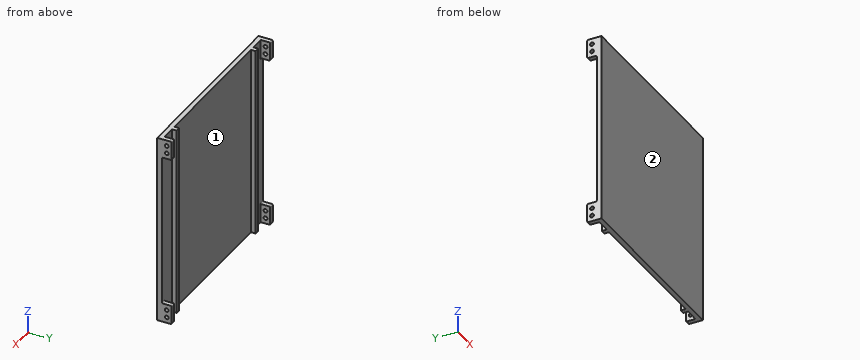
from build123d import *

# Parameters (mm, degrees)
SKETCH1_W            = 200
SKETCH1_H            = 5
BOSS_EXTRUDE1_DEPTH  = 100
SKETCH2_W            = 5
SKETCH2_H            = 200
BOSS_EXTRUDE2_DEPTH  = 5
SKETCH3_W            = 5
SKETCH3_H            = 20
BOSS_EXTRUDE3_DEPTH  = 10
SKETCH4_R            = 2
CUT_EXTRUDE1_DEPTH   = 10
FILLET1_R            = 1
FILLET1_OF_MIRROR1_R = 1


with BuildPart() as part:
    # Sketch1 → Boss-Extrude1 (new, symmetric)
    with BuildSketch(Plane.XY):
        with Locations((0, -2.5)):
            Rectangle(SKETCH1_W, SKETCH1_H)
    extrude(amount=BOSS_EXTRUDE1_DEPTH, both=True)

    # Sketch2 → Boss-Extrude2 (add)
    with BuildSketch(Plane(origin=(0, 0, 0), x_dir=(1, 0, 0), z_dir=(0, 1, 0))):
        with Locations((-78, 0)):
            Rectangle(SKETCH2_W, SKETCH2_H)
        with Locations((78, 0)):
            Rectangle(SKETCH2_W, SKETCH2_H)
    extrude(amount=BOSS_EXTRUDE2_DEPTH)

    # Sketch3 → Boss-Extrude3 (add)
    with BuildSketch(Plane(origin=(0, 0, 0), x_dir=(1, 0, 0), z_dir=(0, 1, 0))):
        with Locations((-97.5, -90)):
            Rectangle(SKETCH3_W, SKETCH3_H)
        with Locations((-97.5, 90)):
            Rectangle(SKETCH3_W, SKETCH3_H)
    boss_extrude3 = extrude(amount=BOSS_EXTRUDE3_DEPTH)

    # Sketch4 → Cut-Extrude1 (cut)
    with BuildSketch(Plane.ZY.offset(100)):
        with Locations((-86, 5)):
            Circle(SKETCH4_R)
        with Locations((-94, 5)):
            Circle(SKETCH4_R)
        with Locations((94, 5)):
            Circle(SKETCH4_R)
        with Locations((86, 5)):
            Circle(SKETCH4_R)
        with Locations((-86, 5)):
            Circle(SKETCH4_R)
        with Locations((-94, 5)):
            Circle(SKETCH4_R)
    cut_extrude1 = extrude(amount=-CUT_EXTRUDE1_DEPTH, mode=Mode.SUBTRACT)

    # Fillet1
    fillet1_edges = [part.edges().sort_by_distance(p)[0] for p in [
        (-97.5, 0, 80),
        (-97.5, 10, 100),
        (-97.5, 10, 80),
        (-97.5, 0, -80),
        (-97.5, 10, -100),
        (-97.5, 10, -80),
    ]]
    fillet(fillet1_edges, radius=FILLET1_R)

    # Mirror1: Boss-Extrude3, Cut-Extrude1 across plane
    add(boss_extrude3.mirror(Plane(origin=(0, 0, 0), x_dir=(0, 0, 1), z_dir=(1, 0, 0))))
    add(cut_extrude1.mirror(Plane(origin=(0, 0, 0), x_dir=(0, 0, 1), z_dir=(1, 0, 0))), mode=Mode.SUBTRACT)

    # Fillet1 of Mirror1
    fillet1_of_mirror1_edges = [part.edges().sort_by_distance(p)[0] for p in [
        (97.5, 0, 80),
        (97.5, 10, 100),
        (97.5, 10, 80),
        (97.5, 0, -80),
        (97.5, 10, -100),
        (97.5, 10, -80),
    ]]
    fillet(fillet1_of_mirror1_edges, radius=FILLET1_OF_MIRROR1_R)


solid = part.part
Input: part model. Units: mm. Frame: model coordinates. Face numbers are marked on the shaded views. Coordinates: 2 decimals unless noted, no trailing zeros. Order: outer loops, then holes, each group sorted by start corner. A loop starts at its lowest first (then second) coordinate and runs counter-clockwise, first axis right, second up. Notation, with made-up numbers: M -6.75,18.25 L 45.25,18.25 A22 cw 45.25,29.25 Z; hole C -7.75,48 d6. An arc over 180 degrees is marked long. Write item = value, one per line. Start each with the question number.
(1) Pull-direction query (X, two-part tool) for the marked faces 1 and 2; classes: released by +X, released by -X, zero draft, split by the parting line, or undercut.
(2) First-contact query: P1, Ø3.5, axis at y = 5, z = 94, coming from the +X side; P2, Ø2.5, axis at y = 5, z = 94, coming from the -X side; P3, Ø6, axis at x = 15, z = -64.5, coming from the +Y side. Flat tips, straight axial feed; report the tip coordinate or a pass-through.
(3) Section C-C on x = 78. Output: boundary loops of the cut face in (y, z), and give its area (3 significant figures).
(4) Line query: line 1 along X through (y, z) = (2, -82); line 2 along Z through (x, y) = (97.65, 5); line 3 along X through (y, z) = (0.25, 54). Output: solid intervals per line, ascending. Write a range as [from, to].
(5) Section A-A on z = 10. Output: boundary loops of the cut face in (x, y), and give its area (3 significant figures).
(6) Section B-B on x = 53. Output: boundary loops of the cut face in (y, z).
Result set:
q1.face_1 = undercut
q1.face_2 = zero draft
q2.P1 = 80.5
q2.P2 = -80.5
q2.P3 = 0
q3.outline = M -5,-100 L 5,-100 L 5,100 L -5,100 Z
q3.area = 2,000 mm²
q4.line_1 = [-100, -95], [-80.5, -75.5], [75.5, 80.5], [95, 100]
q4.line_2 = [-100, -96], [-92, -88], [-84, -80], [80, 84], [88, 92], [96, 100]
q4.line_3 = [-80.5, -75.5], [75.5, 80.5]
q5.outline = M -100,-5 L 100,-5 L 100,0 L 80.5,0 L 80.5,5 L 75.5,5 L 75.5,0 L -75.5,0 L -75.5,5 L -80.5,5 L -80.5,0 L -100,0 Z
q5.area = 1,050 mm²
q6.outline = M -5,-100 L 0,-100 L 0,100 L -5,100 Z
